```python
from build123d import *

# Parameters (mm, degrees)
EXTRUDE_1_DEPTH = 15


with BuildPart() as part:
    # Model → 凸台-拉伸1 (new body)
    with BuildSketch(Plane.XY):
        Polygon((184.411857588, 120.010493647), (204.418760095, 120.010493647), (204.418760095, 77.010493647), (962.354071701, 130.010493647), (962.354071701, 135.010493647), (912.354071701, 135.010493647), (912.354071701, 155.010493647), (962.354067739, 155.010493647), (962.354063778, 160.010493647), (204.418760095, 213.010493093), (204.411857588, 170.010493647), (184.411857588, 170.010493647), align=None)
        Polygon((258.506130737, 110.010493647), (258.506130737, 180.010493647), (759.029449722, 145.010493647), align=None, mode=Mode.SUBTRACT)
    extrude(amount=EXTRUDE_1_DEPTH)


solid = part.part
```
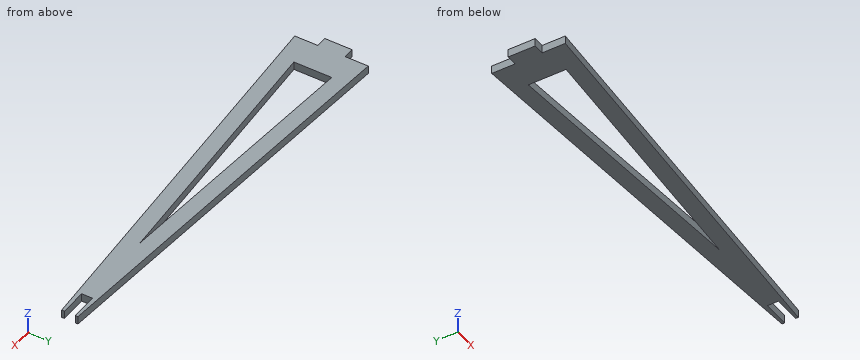
The model under review builds one solid part; all positions refer to its coordinate system, in mm. Give positions to 0.01 mm unless a question says otherwise; leave off trailing zeros. Write each loop counter-clockwise with the first axis right and the second up, starting at its lowest first coordinate (ties: lowest second). Pieces come first, ordered by that corner, then holes.
(1) To check wall thickness, follow L1, parallel to Y at x = 524, z = 10.25; L2, parallel to Y at x = 298, z = 4.75; L3, parallel to Y at x = 766, z = 5. State the ranges of each line that lie inside material, in increasing order.
(2) Consider section A-A, the plane z = 10.5. Give the boundary of the cut face in (x, y).
(3) Consider section C-C, the plane y = 199.5. Give the boundary of the cut face in (x, z), and give its area (3 significant figures).
(4) Consider section D-D, the plane x = 826. Give the boundary of the cut face in (y, z), and give its area (3 significant figures).
(5) Consider section B-B, the plane x = 412. Give the boundary of the cut face in (y, z) (3 decimals), and give its area (3 significant figures).
(6) For P1, Ø5, axis at x = 592, y = 104.5, coming from the -Z side; P2, Ø7.5, axis at y = 141, z = 10.5, coming from the +X side; P3, Ø4.5, axis at x = 197, z = 9.5, coming from the -Y side; P4, Ø1.5, axis at y = 95.5, z = 8.5, coming from the -X side, all flat-tipped, find the tip position at first contact; note any pin that passes through.
Returned:
1. L1: y = 99.36 to 128.58, 161.45 to 190.66
1. L2: y = 83.55 to 112.77, 177.25 to 206.47
1. L3: y = 116.28 to 173.74
2. outline: (184.41, 120.01) - (204.42, 120.01) - (204.42, 77.01) - (962.35, 130.01) - (962.35, 135.01) - (912.35, 135.01) - (912.35, 155.01) - (962.35, 155.01) - (962.35, 160.01) - (204.42, 213.01) - (204.41, 170.01) - (184.41, 170.01) - close; hole (258.51, 110.01) - (759.03, 145.01) - (258.51, 180.01) - close
3. outline: (204.42, 0) - (397.63, 0) - (397.63, 15) - (204.42, 15) - close
3. area: 2,900 mm2
4. outline: (120.48, 0) - (169.55, 0) - (169.55, 15) - (120.48, 15) - close
4. area: 736 mm2
5. outline: (91.526, 0) - (120.744, 0) - (120.744, 15) - (91.526, 15) - close; (169.277, 0) - (198.495, 0) - (198.495, 15) - (169.277, 15) - close
5. area: 877 mm2
6. P1: stops at z = 0
6. P2: stops at x = 912.35
6. P3: stops at y = 120.01
6. P4: stops at x = 204.42
